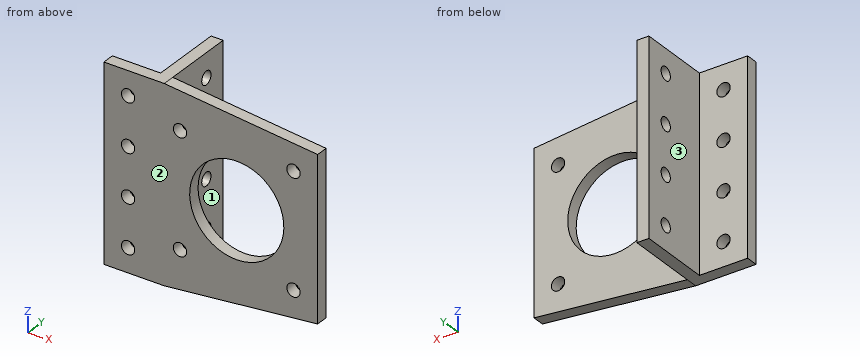
from build123d import *

# Parameters (mm, degrees)
BOSS_EXTRU_1_DEPTH      = 80
ENL_V_MAT_EXTRU_1_REACH = 91.582
ESQUISSE2_R             = 2.75
ENL_V_MAT_EXTRU_2_REACH = 92.436
ESQUISSE3_R             = 2.75
ESQUISSE5_R             = 2.75
ESQUISSE5_R_2           = 19.5
BOSS_EXTRU_2_DEPTH      = 5


with BuildPart() as part:
    # Esquisse1 → Boss.-Extru.1 (new body)
    with BuildSketch(Plane.XY):
        Polygon((-4.641855204, 0), (-4.641855204, 35), (-9.641855204, 35), (-9.641855204, 5), (-29.641855204, 5), (-29.641855204, 0), align=None)
    extrude(amount=BOSS_EXTRU_1_DEPTH)

    # Esquisse2 → Enlèv. mat.-Extru.1 (cut, up to next)
    with BuildSketch(Plane.ZY.offset(9.641855204), mode=Mode.PRIVATE) as enl_v_mat_extru_1_sk1:
        with Locations(Location((10, 25, 0), (0, 0, 270))):
            Circle(ESQUISSE2_R)
    enl_v_mat_extru_1_tool1 = extrude(enl_v_mat_extru_1_sk1.sketch, amount=-ENL_V_MAT_EXTRU_1_REACH, mode=Mode.PRIVATE) & part.part
    # Esquisse2 → Enlèv. mat.-Extru.1 (cut, up to next)
    with BuildSketch(Plane.ZY.offset(9.641855204), mode=Mode.PRIVATE) as enl_v_mat_extru_1_sk2:
        with Locations(Location((50, 25, 0), (0, 0, 270))):
            Circle(ESQUISSE2_R)
    enl_v_mat_extru_1_tool2 = extrude(enl_v_mat_extru_1_sk2.sketch, amount=-ENL_V_MAT_EXTRU_1_REACH, mode=Mode.PRIVATE) & part.part
    # Esquisse2 → Enlèv. mat.-Extru.1 (cut, up to next)
    with BuildSketch(Plane.ZY.offset(9.641855204), mode=Mode.PRIVATE) as enl_v_mat_extru_1_sk3:
        with Locations(Location((70, 25, 0), (0, 0, 270))):
            Circle(ESQUISSE2_R)
    enl_v_mat_extru_1_tool3 = extrude(enl_v_mat_extru_1_sk3.sketch, amount=-ENL_V_MAT_EXTRU_1_REACH, mode=Mode.PRIVATE) & part.part
    # Esquisse2 → Enlèv. mat.-Extru.1 (cut, up to next)
    with BuildSketch(Plane.ZY.offset(9.641855204), mode=Mode.PRIVATE) as enl_v_mat_extru_1_sk4:
        with Locations(Location((30, 25, 0), (0, 0, 270))):
            Circle(ESQUISSE2_R)
    enl_v_mat_extru_1_tool4 = extrude(enl_v_mat_extru_1_sk4.sketch, amount=-ENL_V_MAT_EXTRU_1_REACH, mode=Mode.PRIVATE) & part.part
    add(enl_v_mat_extru_1_tool1.solids().sort_by_distance((-9.641855, 25, 10))[0], mode=Mode.SUBTRACT)
    add(enl_v_mat_extru_1_tool2.solids().sort_by_distance((-9.641855, 25, 50))[0], mode=Mode.SUBTRACT)
    add(enl_v_mat_extru_1_tool3.solids().sort_by_distance((-9.641855, 25, 70))[0], mode=Mode.SUBTRACT)
    add(enl_v_mat_extru_1_tool4.solids().sort_by_distance((-9.641855, 25, 30))[0], mode=Mode.SUBTRACT)

    # Esquisse3 → Enlèv. mat.-Extru.2 (cut, up to next)
    with BuildSketch(Plane(origin=(0, 5, 0), x_dir=(1, 0, 0), z_dir=(0, 1, 0)), mode=Mode.PRIVATE) as enl_v_mat_extru_2_sk1:
        with Locations(Location((-19.641855204, -10, 0), (0, 0, 180))):
            Circle(ESQUISSE3_R)
    enl_v_mat_extru_2_tool1 = extrude(enl_v_mat_extru_2_sk1.sketch, amount=-ENL_V_MAT_EXTRU_2_REACH, mode=Mode.PRIVATE) & part.part
    # Esquisse3 → Enlèv. mat.-Extru.2 (cut, up to next)
    with BuildSketch(Plane(origin=(0, 5, 0), x_dir=(1, 0, 0), z_dir=(0, 1, 0)), mode=Mode.PRIVATE) as enl_v_mat_extru_2_sk2:
        with Locations(Location((-19.641855204, -30, 0), (0, 0, 180))):
            Circle(ESQUISSE3_R)
    enl_v_mat_extru_2_tool2 = extrude(enl_v_mat_extru_2_sk2.sketch, amount=-ENL_V_MAT_EXTRU_2_REACH, mode=Mode.PRIVATE) & part.part
    # Esquisse3 → Enlèv. mat.-Extru.2 (cut, up to next)
    with BuildSketch(Plane(origin=(0, 5, 0), x_dir=(1, 0, 0), z_dir=(0, 1, 0)), mode=Mode.PRIVATE) as enl_v_mat_extru_2_sk3:
        with Locations(Location((-19.641855204, -50, 0), (0, 0, 180))):
            Circle(ESQUISSE3_R)
    enl_v_mat_extru_2_tool3 = extrude(enl_v_mat_extru_2_sk3.sketch, amount=-ENL_V_MAT_EXTRU_2_REACH, mode=Mode.PRIVATE) & part.part
    # Esquisse3 → Enlèv. mat.-Extru.2 (cut, up to next)
    with BuildSketch(Plane(origin=(0, 5, 0), x_dir=(1, 0, 0), z_dir=(0, 1, 0)), mode=Mode.PRIVATE) as enl_v_mat_extru_2_sk4:
        with Locations(Location((-19.641855204, -70, 0), (0, 0, 180))):
            Circle(ESQUISSE3_R)
    enl_v_mat_extru_2_tool4 = extrude(enl_v_mat_extru_2_sk4.sketch, amount=-ENL_V_MAT_EXTRU_2_REACH, mode=Mode.PRIVATE) & part.part
    add(enl_v_mat_extru_2_tool1.solids().sort_by_distance((-19.641855, 5, 10))[0], mode=Mode.SUBTRACT)
    add(enl_v_mat_extru_2_tool2.solids().sort_by_distance((-19.641855, 5, 30))[0], mode=Mode.SUBTRACT)
    add(enl_v_mat_extru_2_tool3.solids().sort_by_distance((-19.641855, 5, 50))[0], mode=Mode.SUBTRACT)
    add(enl_v_mat_extru_2_tool4.solids().sort_by_distance((-19.641855, 5, 70))[0], mode=Mode.SUBTRACT)

    # Esquisse5 → Boss.-Extru.2 (add)
    with BuildSketch(Plane.XZ):
        Polygon((-4.641855204, 0), (58.858144796, 6.5), (58.858144796, 73.5), (-4.641855204, 80), align=None)
        with Locations(Location((1.858144796, 16.5, 0), (0, 0, 270))):
            Circle(ESQUISSE5_R, mode=Mode.SUBTRACT)
        with Locations(Location((1.858144796, 63.5, 0), (0, 0, 270))):
            Circle(ESQUISSE5_R, mode=Mode.SUBTRACT)
        with Locations(Location((48.858144796, 63.5, 0), (0, 0, 270))):
            Circle(ESQUISSE5_R, mode=Mode.SUBTRACT)
        with Locations(Location((48.858144796, 16.5, 0), (0, 0, 270))):
            Circle(ESQUISSE5_R, mode=Mode.SUBTRACT)
        with Locations(Location((25.358144796, 40, 0), (0, 0, 270))):
            Circle(ESQUISSE5_R_2, mode=Mode.SUBTRACT)
    extrude(amount=-BOSS_EXTRU_2_DEPTH)


solid = part.part
Input: part model. Units: mm. Frame: model coordinates. Face numbers are marked on the shaded views. A direction names the side the tool comes from. Coordinates: 2 decimals unless noted, no trailing zeros. Order: outer loops, then holes, each group sorted by start corner. A loop starts at its lowest first (then second) coordinate and runs counter-clockwise, first axis right, second up.
1. Cut plane B-B, the plane z = 16.5. Return loops of the section in (x, y), plus the area to 4 significant figures.
Checked values:
outline: (-29.64, 0) - (-0.89, 0) - (-0.89, 5) - (-4.64, 5) - (-4.64, 35) - (-9.64, 35) - (-9.64, 5) - (-29.64, 5) - close; (4.61, 0) - (46.11, 0) - (46.11, 5) - (4.61, 5) - close; (51.61, 0) - (58.86, 0) - (58.86, 5) - (51.61, 5) - close
area: 537.5 mm2
2. Cut plane C-C, the plane y = 4. Count the separate pieces of the cut face and the enclosed holes in it, plus the area to 3 significant figures.
Checked values:
separate pieces: 1
enclosed holes: 9
area: 5,280 mm2
3. Cut plane D-D, the plane x = 42.5. Return loops of the section in (y, z).
Checked values:
outline: (0, 4.83) - (5, 4.83) - (5, 30.7) - (0, 30.7) - close; (0, 49.3) - (5, 49.3) - (5, 75.17) - (0, 75.17) - close
4. Contact query for flat-ended pins moving along their axis: P1, Ø6.5, axis at y = 25, z = 10, coming from the -X side; P2, Ø12, axis at x = 29, y = 5.5, coming from the -Z side; P3, Ø3, axis at x = 47.5, z = 62, coming from the +Y side. Output: stop coordinate, or through.
Checked values:
P1: stops at x = -9.64
P2: stops at z = 2.83
P3: stops at y = 5
5. Ray query, line 1 along X through (y, z) = (1.85, 63.5); line 2 along Z through (x, y) = (-6.3, 25); line 3 along Y through (x, z) = (2, 11). Return the intervals inside material, ascending.
Checked values:
line 1: x = -29.64 to -0.89, 4.61 to 46.11, 51.61 to 58.86
line 2: z = 0 to 7.25, 12.75 to 27.25, 32.75 to 47.25, 52.75 to 67.25, 72.75 to 80
line 3: y = 0 to 5
6. Access query for the marked faces 1, 2 and 3. Directions: +Z, -Z, +X, -X, +Y, -Y. A direction counts if a zero-diameter tool reaches every point of the face in a straight line with its end or side. Return the directions, or none.
Checked values:
face 1: +Z, -Z, +X, +Y
face 2: +Z, -Z, +X, -X, -Y
face 3: +Z, -Z, -X, +Y
7. Cut plane A-A, the plane z = 40. Return loops of the section in (x, y).
Checked values:
outline: (-29.64, 0) - (5.86, 0) - (5.86, 5) - (-4.64, 5) - (-4.64, 35) - (-9.64, 35) - (-9.64, 5) - (-29.64, 5) - close; (44.86, 0) - (58.86, 0) - (58.86, 5) - (44.86, 5) - close
